Can you work these out from the model? Positions are in its coordinate system, mm. Face numbers are marked on the shaded views. A direction names the side the tool comes from. Round coordinates to 2 decimals unless told otherwise and drop trailing zeros. Loops run counter-clockwise (first coordinate to the right, second up) from the corner with the lowest first, then second, coordinate; pieces in that order, holes last.
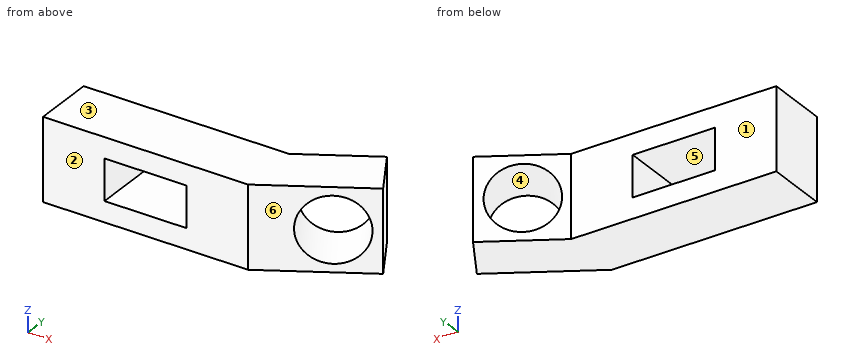
```python
from build123d import *

# Parameters (mm, degrees)
SKETCH_1_W          = 50
SKETCH_1_H          = 20
SKETCH_1_W_2        = 20
SKETCH_1_H_2        = 10
EXTRUDE_1_DEPTH     = 15
EXTRUDE_2_DEPTH     = 20
SKETCH_3_R          = 8
CUT_EXTRUDE_1_DEPTH = 56.775595694


with BuildPart() as part:
    # 草图1 → 凸台-拉伸1 (new body)
    with BuildSketch(Plane(origin=(0, 0, 0), x_dir=(1, 0, 0), z_dir=(0, 1, 0))):
        Rectangle(SKETCH_1_W, SKETCH_1_H)
        Rectangle(SKETCH_1_W_2, SKETCH_1_H_2, mode=Mode.SUBTRACT)
    extrude(amount=EXTRUDE_1_DEPTH)

    # 草图2 → 凸台-拉伸2 (add)
    with BuildSketch(Plane.XY.offset(10)):
        Polygon((25, 15), (42.320508076, 25), (48.815698604, 13.75), (25, 0), align=None)
    extrude(amount=-EXTRUDE_2_DEPTH)

    # 草图3 → 切除-拉伸1 (cut, through all)
    with BuildSketch(Plane(origin=(-0.245190528, 0.424682453, 0), x_dir=(0.8660254037844378, 0.5000000000000017, 0), z_dir=(-0.5000000000000016, 0.8660254037844377, 0))):
        with Locations(Location((39, 0, 0), (0, 0, 180))):
            Circle(SKETCH_3_R)
    extrude(amount=-CUT_EXTRUDE_1_DEPTH, mode=Mode.SUBTRACT)


solid = part.part
```
(1) Suppose I cut it at C-C (z = -1). Write out the boundary of the cut face in (x, y).
(2) We'd pull the mould along Y, two halves only. Please class the marked faces 1, 2, 3 and 4: released by +Y, released by -Y, zero draft, split by the parting line, or undercut.
(3) Suppose I cut it at D-D (x = 12). Write out the boundary of the cut face in (y, z), then the cut area to 3 significant figures.
(4) If I drill on line 1 (Z direction, x = -5.5, y = 13.5); line 2 (Y direction, x = -0.5, z = -5.75); line 3 (X direction, y = 11.5, z = 1), over which ranges is the centre line in solid material (lowest first)?
(5) Suppose I cut it at B-B (z = -4). Give the number of separate pieces and of enclosed holes in the cut face, then the cut area to 3 significant figures.
(6) For pin 1 (10 mm diameter, centred on x = -5, z = -1.5, fed in from +Y); pin 2 (1.5 mm diameter, centred on y = 5.5, z = 2, fed in from +X); pin 3 (4 mm diameter, centred on x = 29.5, z = 7, fed in from +Y), each with a flat end and sliding along its axis, tell me the tip position at first contact or that it passes through.
(7) Which directions (+Z, -Z, +X, -X, +Y, -Y) give clear straight access to the entire face, cutting with the end or side of a thin tool? Please do the marked faces 5 and 6.
(8) Suppose I cut it at A-A (x = -5). Write out the boundary of the cut face in (y, z), then the cut area to 3 significant figures.
Check result:
1. outline: (-25, 0) - (-10, 0) - (-10, 15) - (-25, 15) - close; (10, 0) - (25, 0) - (33.15, 4.71) - (26.66, 15.96) - (25, 15) - (10, 15) - close; (40.4, 23.89) - (46.9, 12.64) - (48.82, 13.75) - (42.32, 25) - close
2. face 1: released by +Y
2. face 2: released by -Y
2. face 3: zero draft
2. face 4: undercut
3. outline: (0, -10) - (15, -10) - (15, 10) - (0, 10) - close
3. area: 300 mm2
4. line 1: z = -10 to -5, 5 to 10
4. line 2: y = 0 to 15
4. line 3: x = -25 to -10, 10 to 29.23
5. separate pieces: 3
5. enclosed holes: 0
5. area: 579 mm2
6. pin 1: stops at y = 15
6. pin 2: stops at x = 33.41
6. pin 3: stops at y = 18.7
7. face 5: +Y, -Y
7. face 6: +Z, -Z, +X, -Y
8. outline: (0, -10) - (15, -10) - (15, -5) - (0, -5) - close; (0, 5) - (15, 5) - (15, 10) - (0, 10) - close
8. area: 150 mm2
